Part print with two shaded views. Sizes in mm from the minimum x, y, z corner. Give positions to 0.01 mm unless a question says otherwise; leave off trailing zeros. Write each loop counter-clockwise with the first axis right and the second up, starting at its lowest first coordinate (ties: lowest second). Pieces come first, ordered by that corner, then holes. Notation, with made-up numbers: (-36, 73.25) -> (-2, 73.25) arc R20 cw to (-2, 92.25) -> close; hole circle Ø9 at (58.5, 36). An arc over 180 degrees is marked (long way). Answer as a JSON object with one key per item and string values.
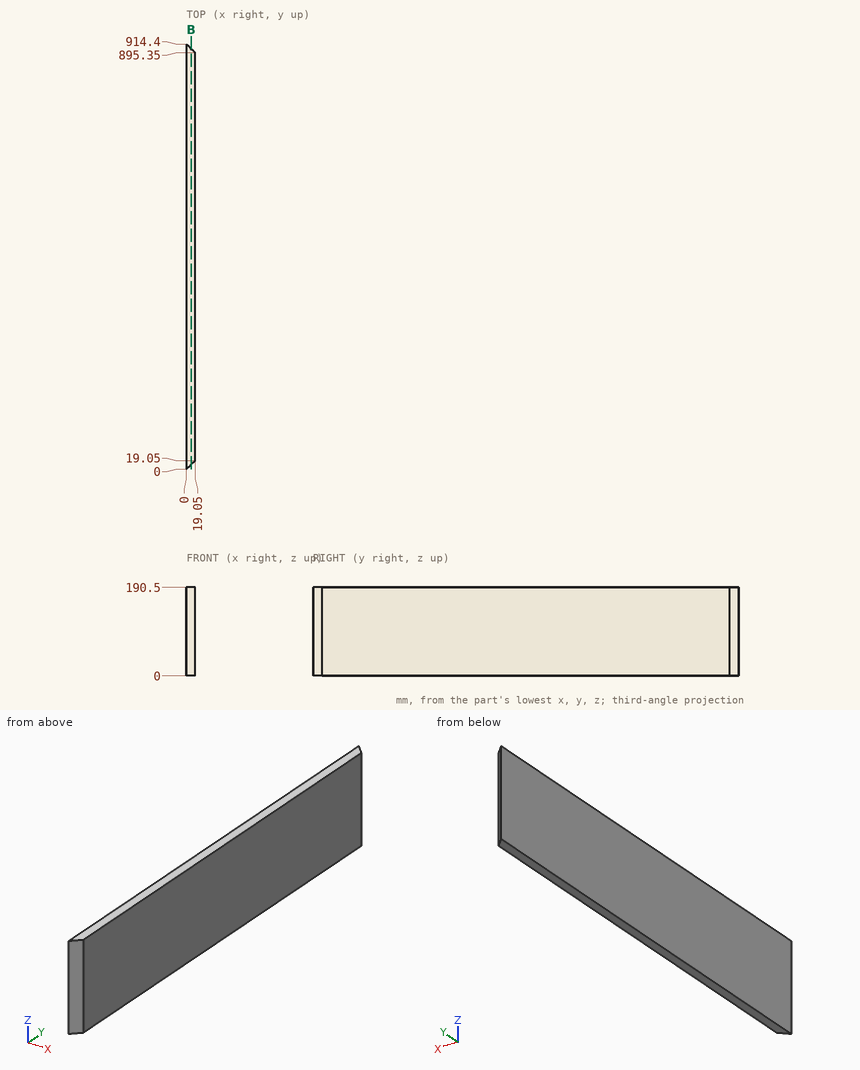
1) Slice it at B-B (x = 10). List the corners of the cut face in (y, z).
Model answer:
{"outline": "(10, 0) -> (904.4, 0) -> (904.4, 190.5) -> (10, 190.5) -> close"}
2) Pin check, flat tips, straight feed: pin 1 (3 mm diameter, centred on x = 4, z = 80, fed in from +Y); pin 2 (6 mm diameter, centred on x = 16.5, y = 313, fed in from -Z); pin 3 (3 mm diameter, centred on x = 10.5, z = 145, fed in from -Y). Stop position of each tip, or through.
Model answer:
{"pin 1": "stops at y = 911.9", "pin 2": "stops at z = 0", "pin 3": "stops at y = 9"}
3) Wall check: probe 1 along Y at (x, z) = (14.5, 36.5); probe 2 along Y at (x, z) = (17.75, 98). Give the ranges that are in metal, low to high.
Model answer:
{"probe 1": "y = 14.5 to 899.9", "probe 2": "y = 17.75 to 896.65"}
